from build123d import *

# Parameters (mm, degrees)
SKETCH1_R                                        = 1.5
BOSS_EXTRUDE1_DEPTH                              = 6
CBORE_FOR_M3_HEX_HEAD_MACHINE_SCREW1_D           = 3.2
CBORE_FOR_M3_HEX_HEAD_MACHINE_SCREW1_DEPTH       = 6
CBORE_FOR_M3_HEX_HEAD_MACHINE_SCREW1_CBORE_D     = 8.4
CBORE_FOR_M3_HEX_HEAD_MACHINE_SCREW1_CBORE_DEPTH = 2.3


with BuildPart() as part:
    # Sketch1 → Boss-Extrude1 (new body)
    with BuildSketch(Plane(origin=(0, 0, 0), x_dir=(1, 0, 0), z_dir=(0, 1, 0))):
        with BuildLine():
            Line((11.5, 10.2), (11.5, 11))
            ThreePointArc((11.5, 11), (9.449747468, 15.949747468), (4.5, 18))
            Line((4.5, 18), (0, 18))
            Line((0, 18), (-35, 16))
            ThreePointArc((-35, 16), (-41, 10), (-35, 4))
            Line((-35, 4), (0, 2))
            Line((0, 2), (4.5, 2))
            ThreePointArc((4.5, 2), (9.449747468, 4.050252532), (11.5, 9))
            Line((11.5, 9), (11.5, 9.8))
            Line((11.5, 9.8), (9.494662869, 9.8))
            ThreePointArc((9.494662869, 9.8), (2, 10), (9.494662869, 10.2))
            Line((9.494662869, 10.2), (11.5, 10.2))
        make_face()
        with Locations(Location((-35, 10, 0), (0, 0, 270))):
            Circle(SKETCH1_R, mode=Mode.SUBTRACT)
        with Locations(Location((-19, 10, 0), (0, 0, 270))):
            Circle(SKETCH1_R, mode=Mode.SUBTRACT)
    extrude(amount=BOSS_EXTRUDE1_DEPTH)

    # CBORE for M3 Hex Head Machine Screw1
    with Locations(Plane(origin=(0, 6, 0), x_dir=(1, 0, 0), z_dir=(0, 1, 0))):
        with Locations((-19, 10), (-35, 10)):
            CounterBoreHole(CBORE_FOR_M3_HEX_HEAD_MACHINE_SCREW1_D / 2, CBORE_FOR_M3_HEX_HEAD_MACHINE_SCREW1_CBORE_D / 2, CBORE_FOR_M3_HEX_HEAD_MACHINE_SCREW1_CBORE_DEPTH, depth=CBORE_FOR_M3_HEX_HEAD_MACHINE_SCREW1_DEPTH)


solid = part.part
Part model, mm, in its own coordinate system. A direction names the side the tool comes from. Give positions to 0.01 mm unless a question says otherwise; leave off trailing zeros. Loops run counter-clockwise (first coordinate to the right, second up) from the corner with the lowest first, then second, coordinate; pieces in that order, holes last.
(1) Band-saw the part on C-C (z = -12.5). Write the cut outline in (x, y).
Return value:
outline: (-40.45, 0) - (2.95, 0) - (2.95, 6) - (-15.63, 6) - (-15.63, 3.7) - (-22.37, 3.7) - (-22.37, 6) - (-31.63, 6) - (-31.63, 3.7) - (-38.37, 3.7) - (-38.37, 6) - (-40.45, 6) - close; (8.55, 0) - (11.34, 0) - (11.34, 6) - (8.55, 6) - close
(2) Pin check, flat tips, straight feed: pin 1 (7.5 mm diameter, centred on x = -19, z = -10, fed in from +Y); pin 2 (1 mm diameter, centred on x = 10.5, y = 2.5, fed in from +Z); pin 3 (1.6 mm diameter, centred on x = 10.5, y = 3, fed in from -Z); pin 4 (2.5 mm diameter, centred on x = -19, z = -10, fed in from -Y). Stop position of each tip, or through.
Return value:
pin 1: stops at y = 3.7
pin 2: stops at z = -4.67
pin 3: stops at z = -15.69
pin 4: passes through
(3) 3-axis set-ups, long thin cutter, end or side, ignore diameter. For faces 4 (the cylindrical face through (-23.196, 4.866, -10.185)), 5 (the flat face through (10, 3, -10.2)), 6 (the flat face through (-9, 6, -10)): which of +Z, -Z, +X, -X, +Y, -Y reach the whole face in a straight line?
Return value:
face 4: +Y
face 5: +X, +Y, -Y
face 6: +Z, -Z, +X, -X, +Y
(4) Drill centre lines: line 1 along X through (y, z) = (2.45, -10); line 2 along Y through (x, z) = (-20, -14); line 3 along Z through (x, y) = (-19, 4.95). Where is each one in solid material? Low to high.
Return value:
line 1: x = -41 to -36.6, -33.4 to -20.6, -17.4 to 2
line 2: y = 0 to 3.7
line 3: z = -16.91 to -14.2, -5.8 to -3.09
(5) Band-saw the part on A-A (x = -35.5). Write the cut outline in (y, z), and give its area (3 significant figures).
Return value:
outline: (0, -15.98) - (6, -15.98) - (6, -14.17) - (3.7, -14.17) - (3.7, -11.52) - (0, -11.52) - close; (0, -8.48) - (3.7, -8.48) - (3.7, -5.83) - (6, -5.83) - (6, -4.02) - (0, -4.02) - close
area: 41.3 mm2
(6) Band-saw the part on B-B (y = 0.7). Write the cut outline in (x, z).
Return value:
outline: (-35, -16) - (0, -18) - (4.5, -18) arc R7 ccw to (11.5, -11) - (11.5, -10.2) - (9.49, -10.2) arc R3.75 cw (long way) to (9.49, -9.8) - (11.5, -9.8) - (11.5, -9) arc R7 ccw to (4.5, -2) - (0, -2) - (-35, -4) arc R6 ccw to start; hole circle Ø3.2 at (-35, -10); hole circle Ø3.2 at (-19, -10)
(7) Band-saw the part on D-D (x = 8). Write the cut outline in (y, z), and give its area (3 significant figures).
Return value:
outline: (0, -17.06) - (6, -17.06) - (6, -13) - (0, -13) - close; (0, -7) - (6, -7) - (6, -2.94) - (0, -2.94) - close
area: 48.7 mm2
(8) Pull direction Z, two halves, no side cores. Call faces 1 (the flat face through (11, 3, -9.8)), 2 (the cylindrical face through (9.4, 3, -4)), 3 (the cylindrical face through (-41, 3, -10)): pulls with the +Z half, pulls with the -Z half, needs draft (parallel to the pull), parting line crosses it, or undercut.
Return value:
face 1: undercut
face 2: pulls with the +Z half
face 3: parting line crosses it
